The model under review builds one solid part; all positions refer to its coordinate system, in mm. A direction names the side the tool comes from. Give positions to 0.01 mm unless a question says otherwise; leave off trailing zeros. Write each loop counter-clockwise with the first axis right and the second up, starting at its lowest first coordinate (ties: lowest second). Pieces come first, ordered by that corner, then holes.
from build123d import *

# Parameters (mm, degrees)
BOX001_W      = 20
BOX001_H      = 20
BOX001_DEPTH  = 320
BOX_W         = 20
BOX_H         = 20
BOX_DEPTH     = 320
SKETCH005_R   = 2.05
HOLE_DEPTH    = 1.501
SKETCH011_R   = 2.05
HOLE006_DEPTH = 1.501
SKETCH013_R   = 2.05
HOLE008_DEPTH = 21.501


with BuildPart() as cut015:
    # Box001 → Box001 (new body)
    with BuildSketch(Plane(origin=(1.5, 1.5, 0), x_dir=(1, 0, 0), z_dir=(0, 0, 1))):
        with Locations((10, 10)):
            Rectangle(BOX001_W, BOX001_H)
    extrude(amount=BOX001_DEPTH)


with BuildPart() as vertical_front_left_body:
    # Box → Box (new body)
    with BuildSketch(Plane.XY):
        with Locations((10, 10)):
            Rectangle(BOX_W, BOX_H)
    extrude(amount=BOX_DEPTH)

    # Cut001: cut Cut015
    add(cut015.part, mode=Mode.SUBTRACT)

    # Sketch005 → Hole (cut, through all)
    with BuildSketch(Plane.YZ.offset(1.5)):
        with Locations((10.75, 28.25)):
            Circle(SKETCH005_R)
    extrude(amount=-HOLE_DEPTH, mode=Mode.SUBTRACT)

    # Sketch011 → Hole006 (cut, through all)
    with BuildSketch(Plane.YZ.offset(1.5)):
        with Locations((10.75, 178.75)):
            Circle(SKETCH011_R)
    extrude(amount=-HOLE006_DEPTH, mode=Mode.SUBTRACT)

    # Sketch013 → Hole008 (cut, through all)
    with BuildSketch(Plane.XZ.offset(1.5)):
        with Locations((10.75, 259.25)):
            Circle(SKETCH013_R)
        with Locations((11.5, 29.75)):
            Circle(SKETCH013_R)
    extrude(amount=-HOLE008_DEPTH, mode=Mode.SUBTRACT)


with BuildPart() as vertical_front_left_mirror:
    # Part__Mirroring002: instance of vertical_front_left_body
    add(vertical_front_left_body.part.mirror(Plane(origin=(0, 0, 0), x_dir=(0, -1, 0), z_dir=(1, 0, 0))))


with BuildPart() as vertical_front_left_mirror_1:
    # Part__Mirroring002 placement: moved
    add(vertical_front_left_mirror.part.moved(Location((640, 0, 0))))


solid = vertical_front_left_mirror_1.part
1) To check wall thickness, follow probe 1 along Z at (x, y) = (639.3, 10.75); probe 2 along X at (y, z) = (0.75, 259.25); probe 3 along Z at (x, y) = (628.5, 0.95). State the ranges of each line that lie inside material, in increasing order.
2) Consider section A-A, the plane z = 95. Give the boundary of the cut face in (x, y), then the cut area to 4 significant figures.
3) Consider section C-C, the plane y = 16.5. Give the boundary of the cut face in (x, z), then the cut area to 3 significant figures.
4) Consider section B-B, the plane x = 623.75. Give the boundary of the cut face in (y, z), then the cut area to 3 significant figures.
5) Insertion check: pin 1 (6 mm diameter, centred on x = 637.5, y = 3, fed in from -Z); pin 2 (2.5 mm diameter, centred on y = 10.75, z = 178.75, fed in from -X); pin 3 (5.5 mm diameter, centred on y = 10.75, z = 28.25, fed in from -X); pin 4 (9 mm diameter, centred on x = 627, z = 114.5, fed in from +Y). Each pin has a flat end and moves straight along its axis. Give the tip position at first contact, or say it passes through.
6) Tool access review of faces 1 (the flat face through (639, 6, 0)), 2 (the flat face through (638.5, 11, 158)): name each direction out of +Z, -Z, +X, -X, +Y, -Y from which nothing blocks a thin tool from reaching the whole face with its end or side.
Answer block:
1. probe 1: z = 0 to 26.2, 30.3 to 176.7, 180.8 to 320
1. probe 2: x = 620 to 627.2, 631.3 to 640
1. probe 3: z = 0 to 27.7, 31.8 to 257.34, 261.16 to 320
2. outline: (620, 0) - (640, 0) - (640, 20) - (638.5, 20) - (638.5, 1.5) - (620, 1.5) - close
2. area: 57.75 mm2
3. outline: (638.5, 0) - (640, 0) - (640, 320) - (638.5, 320) - close
3. area: 480 mm2
4. outline: (0, 0) - (1.5, 0) - (1.5, 320) - (0, 320) - close
4. area: 480 mm2
5. pin 1: stops at z = 0
5. pin 2: passes through
5. pin 3: stops at x = 638.5
5. pin 4: stops at y = 1.5
6. face 1: -Z, +X, -X, +Y, -Y
6. face 2: +Z, -Z, -X, +Y
